Verification items for the finished model (mm, model axes). A direction names the side the tool comes from. Round coordinates to 2 decimals unless told otherwise and drop trailing zeros. Write each loop counter-clockwise with the first axis right and the second up, starting at its lowest first coordinate (ties: lowest second). Pieces come first, ordered by that corner, then holes. Notation, with made-up numbers: M 56.25,26.5 L 63.25,26.5 A20 cw 63.25,58.5 Z; hole C 69.5,3.25 d5. An arc over 180 degrees is marked long. Answer in a Markdown table with one row per item. Add a question column.
1. Go/stop test with flat-tipped pins: pin 1 Ø1.5 at (x, z) = (6, -8.5) entering from -Y; pin 2 Ø3.5 at (y, z) = (-6.5, -11) entering from -X; pin 3 Ø3 at (x, y) = (9, -9) entering from +Z. Record where each tip stops, or that it passes through.
2. Sectioned sample at A-A on y = -7. Record the cut outline in (x, z), plus the area to 3 significant figures.
3. Draft check along Z on faces 4 (the flat face through (2, -8, -7)), 5 (the flat face through (7, -7, -22)), 6 (the flat face through (1, -8, -16.5)). Enter one of: pulls with the +Z half, pulls with the -Z half, needs draft (parallel to the pull), parting line crosses it, or undercut.
4. Sectioned sample at C-C on x = 11.5. Record the cut outline in (y, z), plus the area to 3 significant figures.
5. Set-up check for faces 1 (the flat face through (12, -8, -10)), 2 (the flat face through (1, -8, -13.5)), 3 (the flat face through (0, -7, -11)): record each of +Z, -Z, +X, -X, +Y, -Y from which the full face is reachable in a straight line by a thin tool's end or side.
6. Sectioned sample at B-B on z = -10.25. Record the cut outline in (x, y).
7. Material ranges on probe 1 along X at (y, z) = (-11.5, -2.75); probe 2 along Y at (x, z) = (8.5, -19.5); probe 3 along Z at (x, y) = (8.5, -9.75), recorded low to high.
Autodesk Inventor part; units mm, degrees
ref_plane "YZ Plane" through (0, 0, 0) normal (1, 0, 0) x (0, 1, 0)
ref_plane "XZ Plane" through (0, 0, 0) normal (0, 1, 0) x (-1, 0, 0)
ref_plane "XY Plane" through (0, 0, 0) normal (0, 0, 1) x (1, 0, 0)
sketch "Sketch1" plane through (0, 0, 0) normal (0, 0, 1) x (1, 0, 0)
  line L0 (0, 0) -> (14, 0)
  line L1 (14, 0) -> (14, -14)
  line L2 (14, -14) -> (0, -14)
  line L3 (0, -14) -> (0, 0)
  dimension "d0" = 14
  dimension "d1" = 14
extrude "Extrusion1" add sketch "Sketch1" against normal blind 22
sketch "Sketch2" plane through (0, 0, 0) normal (0, 0, 1) x (1, 0, 0)
  line L0 (2, -2) -> (12, -2)
  line L1 (12, -2) -> (12, -22)
  line L2 (12, -22) -> (2, -22)
  line L3 (2, -22) -> (2, -2)
  point P0 (0, 0)
  dimension "d4" = 10
  dimension "d5" = 20
extrude "Extrusion2" cut sketch "Sketch2" against normal blind 20
sketch "Sketch3" plane through (0, -14, 0) normal (-1, 0, 0) x (0, 0, 1)
  line L0 (0, 0) -> (-20, 0)
  line L1 (-13.5, 12) -> (-16.5, 12)
  line L2 (-16.5, 12) -> (-16.5, 0)
  line L3 (-16.5, 0) -> (-13.5, 0)
  line L4 (-13.5, 0) -> (-13.5, 12)
  point P0 (0, 14)
  dimension "d8" = 3
extrude "Extrusion3" cut sketch "Sketch3" against normal blind 10
properties part number "housing_v02"
Geometry check:
| question | item | result |
|---|---|---|
| 1 | pin 1 | stops at y = -2 |
| 1 | pin 2 | stops at x = 0 |
| 1 | pin 3 | stops at z = -20 |
| 2 | outline | M 0,-22 L 14,-22 L 14,0 L 12,0 L 12,-20 L 2,-20 L 2,-16.5 L 0,-16.5 Z; M 0,-13.5 L 2,-13.5 L 2,0 L 0,0 Z |
| 2 | area | 102 mm2 |
| 3 | face 4 | needs draft |
| 3 | face 5 | pulls with the -Z half |
| 3 | face 6 | undercut |
| 4 | outline | M -14,-22 L 0,-22 L 0,0 L -2,0 L -2,-20 L -14,-20 Z |
| 4 | area | 68.0 mm2 |
| 5 | face 1 | +Z, -Y |
| 5 | face 2 | -X, -Y |
| 5 | face 3 | +Z, -Z, -X, +Y, -Y |
| 6 | outline | M 0,-14 L 2,-14 L 2,-2 L 12,-2 L 12,-14 L 14,-14 L 14,0 L 0,0 Z |
| 7 | probe 1 | x = 0 to 2, 12 to 14 |
| 7 | probe 2 | y = -2 to 0 |
| 7 | probe 3 | z = -22 to -20 |
